Here's the drawing with two shaded views (mm, measured from the low corner). I have some questions. Give positions to 0.01 mm unless a question says otherwise; leave off trailing zeros. Loops run counter-clockwise (first coordinate to the right, second up) from the corner with the lowest first, then second, coordinate; pieces in that order, holes last. Notation, with made-up numbers: (-28, 25.5) - (28, 25.5) arc R24 cw to (28, 43.5) - close; hole circle Ø6 at (46.5, 68.25). An arc over 180 degrees is marked (long way). Answer as a JSON object with one key per item and string values. Group by question number.
Item 1: Please list where these lines run through material, in increasing order: L1, parallel to Y at x = 10.5, z = 2.1; L2, parallel to Y at x = 11, z = 2.5 (1 decimal); L3, parallel to X at y = 19, z = 2.1.
Item 2: Suppose I cut it at D-D on x = 22.5. Write out the boundary of the cut face in (y, z).
Item 3: Suppose I cut it at B-B on z = 1.5. Write out the boundary of the cut face in (x, y).
Item 4: Will this pin go through, and if not, where does the flat tip stop? pin 1 (1.5 mm diameter, centred on x = 28.5, z = 0.5, fed in from +Y).
Item 5: Suppose I cut it at A-A on x = 10.5. Write out the boundary of the cut face in (y, z).
Item 6: Suppose I cut it at C-C on y = 7.5. Write out the boundary of the cut face in (x, z) (1 decimal).
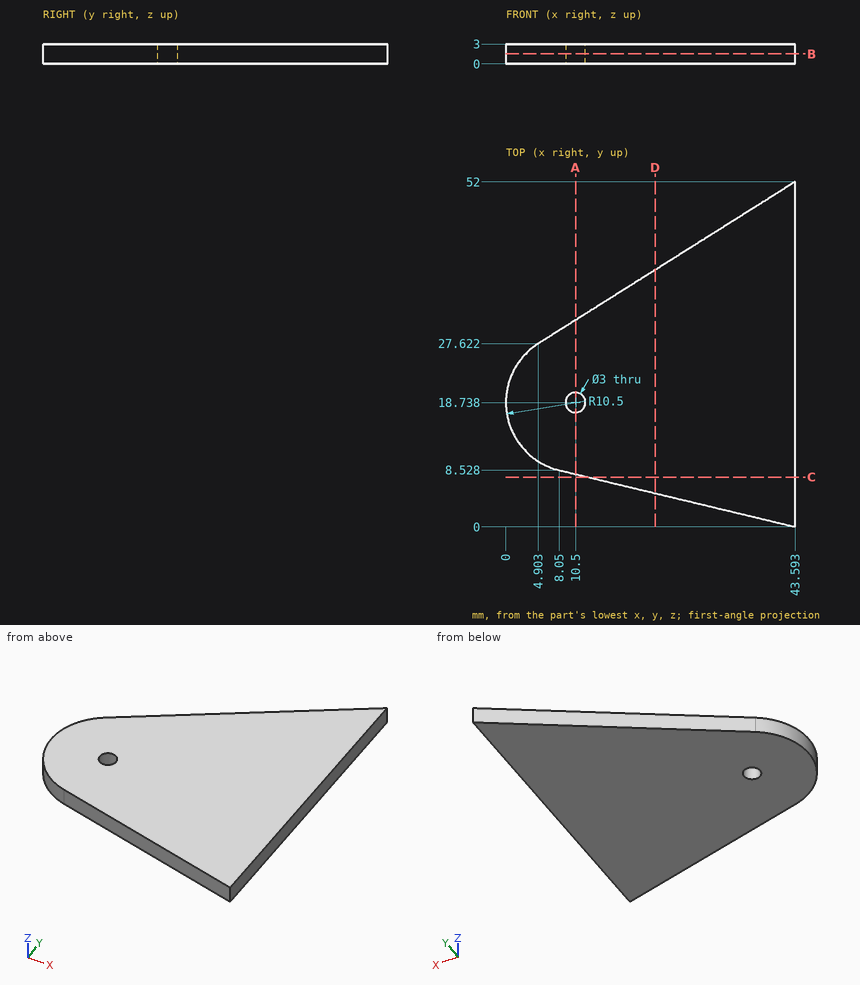
Worked out:
{
 "1": {"L1": "y = 7.94 to 17.24, 20.24 to 31.15", "L2": "y = 7.8 to 17.3, 20.2 to 31.5", "L3": "x = 0 to 9.02, 11.98 to 43.59"},
 "2": {"outline": "(5.06, 0) - (38.71, 0) - (38.71, 3) - (5.06, 3) - close"},
 "3": {"outline": "(4.9, 27.62) arc R10.5 ccw to (8.05, 8.53) - (43.59, 0) - (43.59, 52) - close; hole circle Ø3 at (10.5, 18.74)"},
 "4": {"pin 1": "stops at y = 42.96"},
 "5": {"outline": "(7.94, 0) - (17.24, 0) - (17.24, 3) - (7.94, 3) - close; (20.24, 0) - (31.15, 0) - (31.15, 3) - (20.24, 3) - close"},
 "6": {"outline": "(12.3, 0) - (43.6, 0) - (43.6, 3) - (12.3, 3) - close"}
}
